Read the model definition and answer for the solid it produces. Units are mm, in the model's axes. Face numbers are marked on the shaded views. A direction names the side the tool comes from. Coordinates: 2 decimals unless noted, no trailing zeros. Write each loop counter-clockwise with the first axis right and the second up, starting at its lowest first coordinate (ties: lowest second). Pieces come first, ordered by that corner, then holes. Notation, with made-up numbers: (69, 67.5) -> (103, 67.5) arc R15 ccw to (103, 73.5) -> close; hole circle Ø8 at (32, -13). An arc over 180 degrees is marked (long way). Answer as a JSON object with one key per item and string values. Group by question number.
(1) Flat-ended cylindrical pins translate along their axes: P1, Ø8, axis at x = 37.96, y = 2.68, coming from the -Z side; P2, Ø6, axis at x = 44.5, y = 15.5, coming from the -Z side; P3, Ø6, axis at y = -3, z = -37.5, coming from the +X side. Find the tip coordinate at first contact, or state that the pin passes through.
(2) Find section A-A (y = -10.5). Give the vertices of the cut face in (x, z), then the cut area to 3 significant figures.
(3) Find section D-D (z = -38). Give the vertices of the cut face in (x, y), then the cut area to 3 significant figures.
(4) Find section B-B (z = -43.5). Give the vertices of the cut face in (x, y).
(5) Straight lines are drawn through the part: L1, parallel to Z at x = 22.5, y = -14.5; L2, parallel to X at y = 21.5, z = -31. For each, find the intervals that lie inside material, in ascending order.
(6) Which of the six approach directions +Z, -Z, +X, -X, +Y, -Y give full straight-line access (tool end or side, diameter ignored) to the marked faces 1 and 2?
(7) Find section C-C (x = 12.5). Give the vertices of the cut face in (y, z).
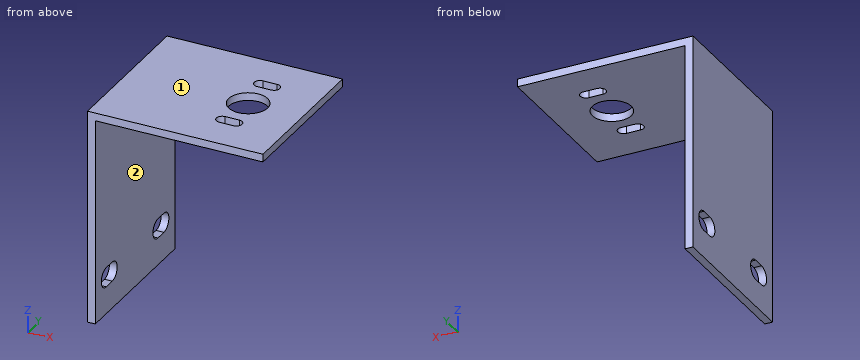
from build123d import *

# Parameters (mm, degrees)
ESQUISSE2_W             = 45
ESQUISSE2_H             = 40
ESQUISSE2_R             = 5
BOSS_EXTRU_8_DEPTH      = 2
ESQUISSE3_W             = 2
ESQUISSE3_H             = 53
BOSS_EXTRU_9_DEPTH      = 40
ENL_V_MAT_EXTRU_1_DEPTH = 40


with BuildPart() as part:
    # Esquisse2 → Boss.-Extru.8 (new body)
    with BuildSketch(Plane.XY):
        with Locations((29.457965055, 2.680327869)):
            Rectangle(ESQUISSE2_W, ESQUISSE2_H)
        with Locations((37.957965055, 2.680327869)):
            Circle(ESQUISSE2_R, mode=Mode.SUBTRACT)
        with BuildLine():
            Line((36.157965055, 13.680327869), (39.757965055, 13.680327869))
            ThreePointArc((39.757965055, 13.680327869), (41.257965055, 12.180327869), (39.757965055, 10.680327869))
            Line((39.757965055, 10.680327869), (36.157965055, 10.680327869))
            ThreePointArc((36.157965055, 10.680327869), (34.657965055, 12.180327869), (36.157965055, 13.680327869))
        make_face(mode=Mode.SUBTRACT)
        with BuildLine():
            Line((36.157965055, -8.319672131), (39.757965055, -8.319672131))
            ThreePointArc((39.757965055, -8.319672131), (41.257965055, -6.819672131), (39.757965055, -5.319672131))
            Line((39.757965055, -5.319672131), (36.157965055, -5.319672131))
            ThreePointArc((36.157965055, -5.319672131), (34.657965055, -6.819672131), (36.157965055, -8.319672131))
        make_face(mode=Mode.SUBTRACT)
    extrude(amount=BOSS_EXTRU_8_DEPTH)

    # Esquisse3 → Boss.-Extru.9 (add)
    with BuildSketch(Plane(origin=(0, 22.680327869, 0), x_dir=(1, 0, 0), z_dir=(0, 1, 0))):
        with Locations((7.957965055, 26.5)):
            Rectangle(ESQUISSE3_W, ESQUISSE3_H)
    extrude(amount=-BOSS_EXTRU_9_DEPTH)

    # Esquisse4 → Enlèv. mat.-Extru.1 (cut)
    with BuildSketch(Plane(origin=(8.957965055, 0, 0), x_dir=(0, 0, -1), z_dir=(1, 0, 0))):
        with BuildLine():
            Line((41, -11.819672131), (41, -8.819672131))
            ThreePointArc((41, -8.819672131), (43.5, -6.319672131), (46, -8.819672131))
            Line((46, -8.819672131), (46, -11.819672131))
            ThreePointArc((46, -11.819672131), (43.5, -14.319672131), (41, -11.819672131))
        make_face()
        with BuildLine():
            Line((41, 17.180327869), (41, 14.180327869))
            ThreePointArc((41, 14.180327869), (43.5, 11.680327869), (46, 14.180327869))
            Line((46, 14.180327869), (46, 17.180327869))
            ThreePointArc((46, 17.180327869), (43.5, 19.680327869), (41, 17.180327869))
        make_face()
    extrude(amount=-ENL_V_MAT_EXTRU_1_DEPTH, mode=Mode.SUBTRACT)


solid = part.part
Results below:
{
 "1": {"P1": "passes through", "P2": "stops at z = 0", "P3": "stops at x = 8.96"},
 "2": {"outline": "(6.96, -53) -> (8.96, -53) -> (8.96, -46) -> (6.96, -46) -> close; (6.96, -41) -> (8.96, -41) -> (8.96, 0) -> (51.96, 0) -> (51.96, 2) -> (6.96, 2) -> close", "area": "186 mm2"},
 "3": {"outline": "(6.96, -17.32) -> (8.96, -17.32) -> (8.96, 22.68) -> (6.96, 22.68) -> close", "area": "80.0 mm2"},
 "4": {"outline": "(6.96, -17.32) -> (8.96, -17.32) -> (8.96, -14.32) -> (6.96, -14.32) -> close; (6.96, -6.32) -> (8.96, -6.32) -> (8.96, 11.68) -> (6.96, 11.68) -> close; (6.96, 19.68) -> (8.96, 19.68) -> (8.96, 22.68) -> (6.96, 22.68) -> close"},
 "5": {"L1": "z = 0 to 2", "L2": "x = 6.96 to 8.96"},
 "6": {"face 1": "+Z, +X, -X, +Y, -Y", "face 2": "-Z, +X, +Y, -Y"},
 "7": {"outline": "(-17.32, 0) -> (22.68, 0) -> (22.68, 2) -> (-17.32, 2) -> close"}
}
